from build123d import *

# Parameters (mm, degrees)
F1_DEPTH = 15.5
F2_DEPTH = 1
F4_D     = 1.8
F4_DEPTH = 4
F4_TIP   = 0.5407745571
F5_D     = 1.8
F5_DEPTH = 4
F5_TIP   = 0.5407745571


with BuildPart() as f1:
    # F0 (on Top) → F1 (new body)
    with BuildSketch(Plane.XY):
        with BuildLine():
            Line((-1, -2.5), (1, -2.5))
            ThreePointArc((1, -2.5), (2.0606601718, -2.0606601718), (2.5, -1))
            Line((2.5, -1), (2.5, 1))
            ThreePointArc((2.5, 1), (2.0606601718, 2.0606601718), (1, 2.5))
            Line((1, 2.5), (-1, 2.5))
            ThreePointArc((-1, 2.5), (-2.0606601718, 2.0606601718), (-2.5, 1))
            Line((-2.5, 1), (-2.5, -1))
            ThreePointArc((-2.5, -1), (-2.0606601718, -2.0606601718), (-1, -2.5))
        make_face()
    extrude(amount=F1_DEPTH)



with BuildPart() as f1b:
    # F0 (on Top) → F1, piece 2 (new body)
    with BuildSketch(Plane.XY):
        with BuildLine():
            Line((4.5, 1), (4.5, -1))
            ThreePointArc((4.5, -1), (4.9393398282, -2.0606601718), (6, -2.5))
            Line((6, -2.5), (8, -2.5))
            ThreePointArc((8, -2.5), (9.0606601718, -2.0606601718), (9.5, -1))
            Line((9.5, -1), (9.5, 1))
            ThreePointArc((9.5, 1), (9.0606601718, 2.0606601718), (8, 2.5))
            Line((8, 2.5), (6, 2.5))
            ThreePointArc((6, 2.5), (4.9393398282, 2.0606601718), (4.5, 1))
        make_face()
    extrude(amount=F1_DEPTH)


with BuildPart() as f1_1:
    add(f1.part)

    add(f1b.part)  # F2 merges F1b
    # F0 (on Top) → F2 (join)
    with BuildSketch(Plane.XY):
        Polygon((2.5, 1), (2.5, -1), (3.5, -1), (4.5, -1), (4.5, 1), (3.5, 1), align=None)
    extrude(amount=F2_DEPTH)

    # F4
    with Locations(Plane.XY.offset(15.5)):
        with Locations((0, 0), (7, 0)):
            Hole(F4_D / 2, depth=F4_DEPTH)
            with Locations((0, 0, -(F4_DEPTH + F4_TIP / 2))):  # 118° drill point
                Cone(0, F4_D / 2, F4_TIP, mode=Mode.SUBTRACT)

    # F5
    with Locations(Plane(origin=(0, 0, 0), x_dir=(1, 0, 0), z_dir=(0, 0, -1))):
        with Locations((7, 0), (0, 0)):
            Hole(F5_D / 2, depth=F5_DEPTH)
            with Locations((0, 0, -(F5_DEPTH + F5_TIP / 2))):  # 118° drill point
                Cone(0, F5_D / 2, F5_TIP, mode=Mode.SUBTRACT)


solid = f1_1.part
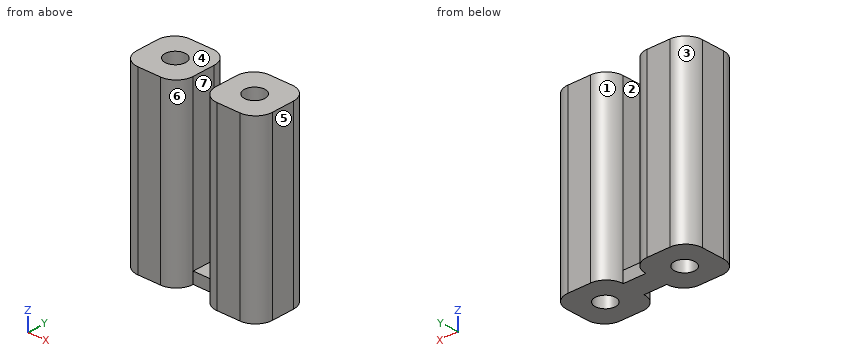
CAD build for the part. Positions are in the model's coordinates, mm. Face numbers are marked on the shaded views. A direction names the side the tool comes from. Round coordinates to 2 decimals unless told otherwise and drop trailing zeros. Write each loop counter-clockwise with the first axis right and the second up, starting at its lowest first coordinate (ties: lowest second). Pieces come first, ordered by that corner, then holes.
(1) Slice it at D-D, the plane x = 1.5. Write the cut outline in (y, z), and give its area (3 significant figures).
(2) Slice it at A-A, the plane z = 8.5. Write the cut outline in (x, y), and give its area (3 significant figures).
(3) 3-axis set-ups, long thin cutter, end or side, ignore diameter. For the marked faces 1, 2 and 3: which of +Z, -Z, +X, -X, +Y, -Y reach the whole face in a straight line?
(4) Slice it at B-B, the plane y = 1.65. Write the cut outline in (x, z), and give its area (3 significant figures).
(5) Probe line 1 along X through (y, z) = (0, 14.2); line 2 along Y through (x, z) = (7, 12.9); line 3 along X through (y, z) = (-2.15, 3.25). List the from-to ranges inside material, lowest first.
(6) Drop flat-ended pins along their axis: P1, Ø1.6, axis at x = 0, y = 0, coming from the -Z side; P2, Ø1.1, axis at x = 7, y = 0, coming from the +Z side; P3, Ø1.4, axis at x = 0, y = 0, coming from the +Z side. Give the stop position or say it passes through.
(7) Slice it at C-C, the plane y = -1.95. Write the cut outline in (x, z), and give its area (3 significant figures).
(8) Mould opens along X. For the marked faces 4, 5, 6 and 7 say: pulls with the +X half, pulls with the -X half, needs draft (parallel to the pull), parting line crosses it, or undercut.
From the geometry:
1. outline: (-2.41, 0) - (2.41, 0) - (2.41, 15.5) - (-2.41, 15.5) - close
1. area: 74.8 mm2
2. outline: (-2.5, -1) arc R1.5 ccw to (-1, -2.5) - (1, -2.5) arc R1.5 ccw to (2.5, -1) - (2.5, 1) arc R1.5 ccw to (1, 2.5) - (-1, 2.5) arc R1.5 ccw to (-2.5, 1) - close; (4.5, -1) arc R1.5 ccw to (6, -2.5) - (8, -2.5) arc R1.5 ccw to (9.5, -1) - (9.5, 1) arc R1.5 ccw to (8, 2.5) - (6, 2.5) arc R1.5 ccw to (4.5, 1) - close
2. area: 46.1 mm2
3. face 1: +Z, -Z, +Y
3. face 2: +Z, +Y, -Y
3. face 3: +Z, -Z, -X, +Y
4. outline: (-2.35, 0) - (2.35, 0) - (2.35, 15.5) - (-2.35, 15.5) - close; (4.65, 0) - (9.35, 0) - (9.35, 15.5) - (4.65, 15.5) - close
4. area: 146 mm2
5. line 1: x = -2.5 to -0.9, 0.9 to 2.5, 4.5 to 6.1, 7.9 to 9.5
5. line 2: y = -2.5 to -0.9, 0.9 to 2.5
5. line 3: x = -1.96 to 1.96, 5.04 to 8.96
6. P1: stops at z = 4.06
6. P2: stops at z = 11.29
6. P3: stops at z = 11.38
7. outline: (-2.16, 0) - (2.16, 0) - (2.16, 15.5) - (-2.16, 15.5) - close; (4.84, 0) - (9.16, 0) - (9.16, 15.5) - (4.84, 15.5) - close
7. area: 134 mm2
8. face 4: needs draft
8. face 5: pulls with the +X half
8. face 6: undercut
8. face 7: undercut
